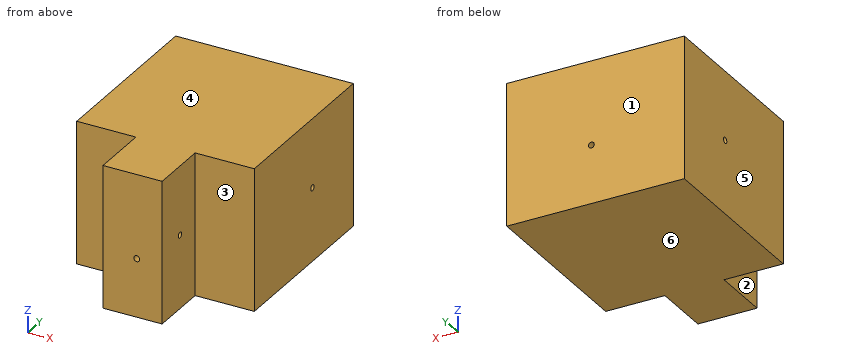
from build123d import *

# Parameters (mm, degrees)
F1_DEPTH = 12
F2_R     = 0.25
F3_DEPTH = 52.1
F4_R     = 0.25
F5_DEPTH = 44
F6_R     = 0.25
F7_DEPTH = 57


with BuildPart() as f1:
    # F0 (on Top) → F1 (new body)
    with BuildSketch(Plane.XY):
        Polygon((0, 20), (-15, 20), (-15, 5), (-10, 5), (-10, 0), (-5, 0), (-5, 5), (0, 5), align=None)
    extrude(amount=F1_DEPTH)

    # F2 (on Right) → F3 (cut)
    with BuildSketch(Plane.YZ):
        with Locations((13.81054, 6.187139)):
            Circle(F2_R)
    extrude(amount=-F3_DEPTH, mode=Mode.SUBTRACT)

    # F4 (on Front) → F5 (cut)
    with BuildSketch(Plane.XZ):
        with Locations((-7.144658, 4.92007)):
            Circle(F4_R)
    extrude(amount=-F5_DEPTH, mode=Mode.SUBTRACT)

    # F6 (on Right) → F7 (cut)
    with BuildSketch(Plane.YZ):
        with Locations((2.697288, 6.192037)):
            Circle(F6_R)
    extrude(amount=-F7_DEPTH, mode=Mode.SUBTRACT)


solid = f1.part
For this review, take the finished solid that the model builds, in its own axes (mm). Face numbers are marked on the shaded views. A direction names the side the tool comes from. Give positions to 0.01 mm unless a question says otherwise; leave off trailing zeros. Loops run counter-clockwise (first coordinate to the right, second up) from the corner with the lowest first, then second, coordinate; pieces in that order, holes last. Notation, with made-up numbers: M 20,70.25 L 29,70.25 A17 ccw 29,89.25 Z; hole C -9,78 d8. An arc over 180 degrees is marked long. Answer as a JSON object with one key per item and string values. Group by question number.
Q1. Add section A-A on z = 7.25. Give the boundary of the cut face in (x, y), and give its area (3 significant figures).
Q2. Add section B-B on x = -10.5. Give the boundary of the cut face in (y, z), and give its area (3 significant figures).
Q3. For probe 1 along X at (y, z) = (3, 7.5); probe 2 along Y at (x, z) = (-5.25, 6.25); probe 3 along Y at (x, z) = (-1.5, 10), list the stretches that pass through material, from the lowest coordinate up. Write a range as [from, to].
Q4. Tool access review of the marked faces 1, 2 and 3: name each direction out of +Z, -Z, +X, -X, +Y, -Y from which nothing blocks a thin tool from reaching the whole face with its end or side.
Q5. Add section C-C on y = 2. Give the boundary of the cut face in (x, z), and give its area (3 significant figures).
Q6. Mouldability with a two-part tool opening along Z and no side actions: class the marked faces 4, 5 and 6 as +Z half, -Z half, draft (parallel to the pull), parting line (faces both ways), or undercut.
Q7. Insertion check: P1, Ø2.5, axis at y = 2, z = 5, coming from the +X side; P2, Ø2.5, axis at x = -1.5, z = 8.5, coming from the -Y side; P3, Ø1, axis at x = -5.5, y = 17, coming from the -Z side. Each pin has a flat end and moves straight along its axis. Give the tip position at first contact, or say it passes through.
Checked values:
{
 "1": {"outline": "M -15,5 L -10,5 L -10,0 L -5,0 L -5,5 L 0,5 L 0,20 L -15,20 Z", "area": "250 mm²"},
 "2": {"outline": "M 5,0 L 20,0 L 20,12 L 5,12 Z; hole C 13.81,6.19 d0.5", "area": "180 mm²"},
 "3": {"probe 1": "[-10, -5]", "probe 2": "[0, 2.45], [2.94, 13.57], [14.05, 20]", "probe 3": "[5, 20]"},
 "4": {"face 1": "+Z, -Z, +X, -X, +Y", "face 2": "+Z, -Z, -X, -Y", "face 3": "+Z, -Z, +X, -Y"},
 "5": {"outline": "M -10,0 L -5,0 L -5,12 L -10,12 Z; hole C -7.14,4.92 d0.5", "area": "59.8 mm²"},
 "6": {"face 4": "+Z half", "face 5": "draft", "face 6": "-Z half"},
 "7": {"P1": "x = -5", "P2": "y = 5", "P3": "z = 0"}
}
